Check sheet for the modelled part. Datum: model origin and axes. Units: mm. Face numbers are marked on the shaded views. A direction names the side the tool comes from. Coordinates: 2 decimals unless noted, no trailing zeros. Loops run counter-clockwise (first coordinate to the right, second up) from the corner with the lowest first, then second, coordinate; pieces in that order, holes last. Notation, with made-up numbers: (61.5, 18.5) - (69.5, 18.5) arc R8 cw to (69.5, 26.5) - close; hole circle Ø8 at (-12.5, 31.25). An arc over 180 degrees is marked (long way). Use a Markdown table: item, result. Add a question column.
1) Sectioned sample at B-B, the plane x = -1.75. Enter the section's corners in (y, z).
2) Sectioned sample at C-C, the plane y = 8.5. Enter the section's corners in (x, z), then the cut area to 3 significant figures.
3) Tool access check on the marked faces 1 and 2. Record the directions out of +Z, -Z, +X, -X, +Y, -Y that give a thin tool (end or side, any length) a straight path to the whole face; none if there is none.
4) Go/stop test with flat-tipped pins: P1, Ø3.5, axis at x = 3.22, z = -66.75, coming from the -Y side; P2, Ø6, axis at x = 1.5, z = -51, coming from the +Y side; P3, Ø6, axis at y = 8, z = -51.5, coming from the +X side. Record where each tip stops, or that it passes through.
5) Thickness scan on line 1 (X direction, y = 8.75, z = -69); line 2 (Y direction, x = -2, z = -49.5). Record the ranges inside material, lowest first.
6) Sectioned sample at A-A, the plane z = -30.5. Enter the section's corners in (x, y).
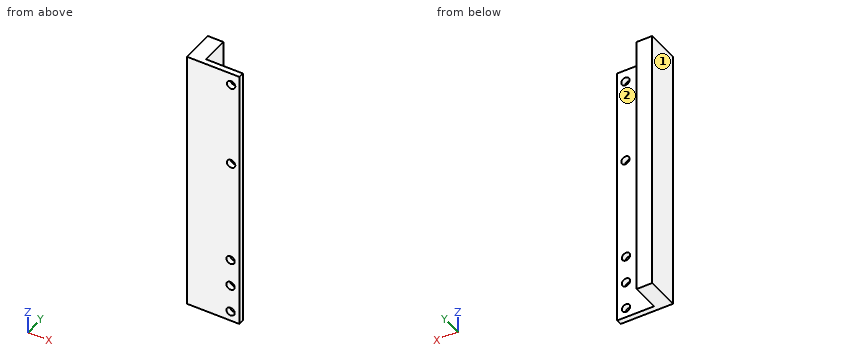
Autodesk Inventor part; units mm, degrees
ref_plane "YZ Plane" through (0, 0, 0) normal (1, 0, 0) x (0, 1, 0)
ref_plane "XZ Plane" through (0, 0, 0) normal (0, 1, 0) x (-1, 0, 0)
ref_plane "XY Plane" through (0, 0, 0) normal (0, 0, 1) x (1, 0, 0)
sketch "Sketch1" plane through (0, 0, 0) normal (0, 1, 0) x (-1, 0, 0)
  line L0 (12.3827, 15.7347) -> (-6.4173, 15.7347)
  line L1 (-6.4173, 15.7347) -> (-6.4173, -80.2653)
  line L2 (-6.4173, -80.2653) -> (12.3827, -80.2653)
  line L3 (12.3827, -80.2653) -> (12.3827, 15.7347)
  circle A0 centre (-3.4173, 11.3847) radius 1.5
  circle A1 centre (-3.4173, -19.2653) radius 1.5
  circle A2 centre (-3.2173, -76.7547) radius 1.5
  circle A3 centre (-3.2173, -66.7547) radius 1.5
  circle A4 centre (-3.2173, -56.7547) radius 1.5
  point P0 (0, 0)
  dimension "d0" = 3
  dimension "d1" = 18.8
  dimension "d2" = 96
  dimension "d3" = 3
  dimension "d4" = 30.65
  dimension "d5" = 35
  dimension "d6" = 3
  dimension "d7" = 3
  dimension "d8" = 3
  dimension "d9" = 3
  dimension "d10" = 3
  dimension "d11" = 10
  dimension "d12" = 10
  dimension "d13" = 3.2
extrude "Extrusion1" add sketch "Sketch1" along normal blind 2
sketch "Sketch2" plane through (0, 2, 0) normal (0, 1, 0) x (1, 0, 0)
  line L0 (6.4173, 80.2653) -> (-12.3827, 80.2653)
  line L1 (-12.3827, -15.7347) -> (6.4173, -15.7347)
  line L2 (-12.3827, 80.2653) -> (-6.7885, 80.2653)
  line L3 (-6.7885, 80.2653) -> (-6.7885, -15.7347)
  line L4 (-6.7885, -15.7347) -> (-12.3827, -15.7347)
  line L5 (-12.3827, -15.7347) -> (-12.3827, 80.2653)
  point P0 (0, 0)
extrude "Extrusion2" add sketch "Sketch2" along normal blind 10
properties part number "connectStepper"
Solved:
| question | item | result |
|---|---|---|
| 1 | outline | (0, -80.27) - (2, -80.27) - (2, 15.73) - (0, 15.73) - close |
| 2 | outline | (-12.38, -80.27) - (-6.79, -80.27) - (-6.79, 15.73) - (-12.38, 15.73) - close |
| 2 | area | 537 mm2 |
| 3 | face 1 | +Z, -Z, -X, +Y, -Y |
| 3 | face 2 | +Z, -Z, +X, +Y |
| 4 | P1 | stops at y = 0 |
| 4 | P2 | stops at y = 2 |
| 4 | P3 | stops at x = -6.79 |
| 5 | line 1 | x = -12.38 to -6.79 |
| 5 | line 2 | y = 0 to 2 |
| 6 | outline | (-12.38, 0) - (6.42, 0) - (6.42, 2) - (-6.79, 2) - (-6.79, 12) - (-12.38, 12) - close |
